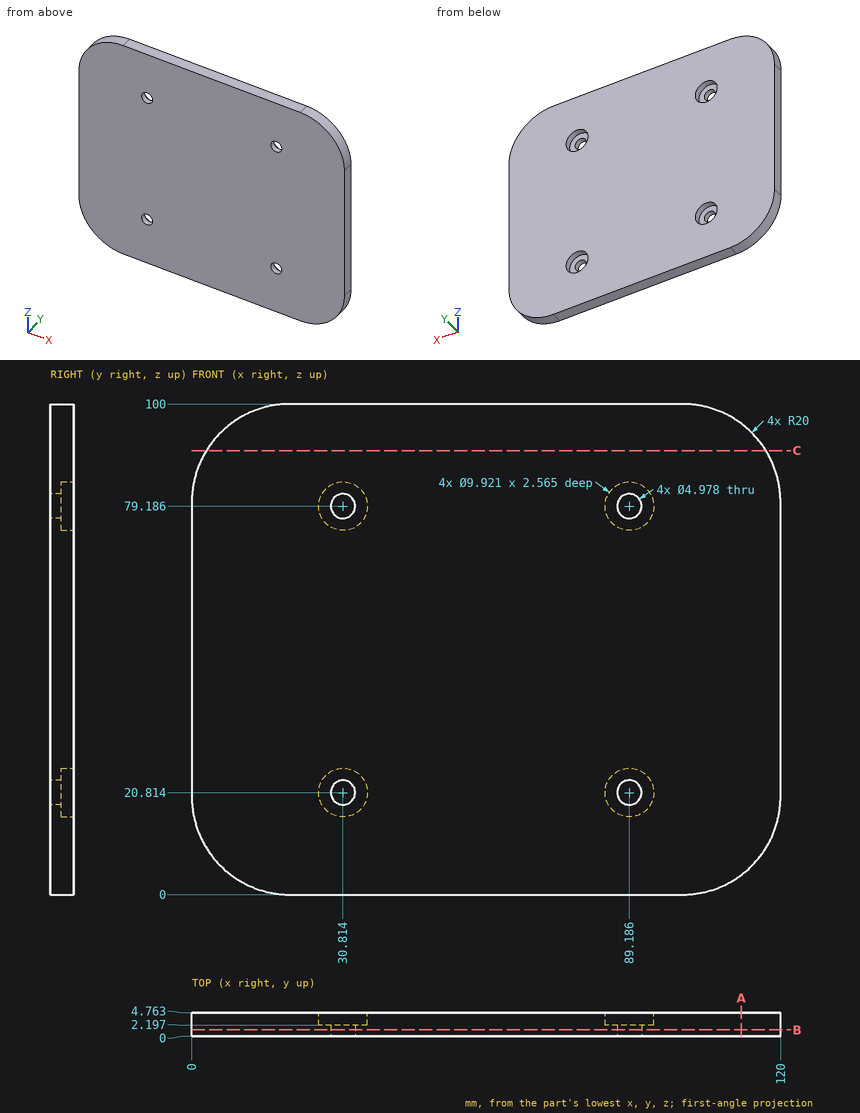
Could you check a few things on this drawing? It's one solid part, dimensions in mm from its lowest x, y, z. Give positions to 0.01 mm unless a question says otherwise; leave off trailing zeros. Write each loop counter-clockwise with the first axis right and the second up, starting at its lowest first coordinate (ties: lowest second). Pieces come first, ordered by that corner, then holes.
(1) Imagine slicing it at C-C, the plane z = 90.5. Write out the boundary of the cut face in (x, y), and give its area (3 significant figures).
Output values:
outline: (2.98, 0) - (117.02, 0) - (117.02, 4.76) - (2.98, 4.76) - close
area: 543 mm2
(2) Imagine slicing it at A-A, the plane x = 112. Write out the boundary of the cut face in (y, z), and give its area (3 significant figures).
Output values:
outline: (0, 4) - (4.76, 4) - (4.76, 96) - (0, 96) - close
area: 438 mm2
(3) If I drill on L1, parallel to X at y = 4, z = 81 (1 decimal); L2, parallel to Z at x = 88, y = 2.3; L3, parallel to X at y = 2.05, z = 91.5 (1 decimal), over which ranges is the centre line in solid material (lowest first)?
Output values:
L1: x = 0 to 26.2, 35.4 to 84.6, 93.8 to 120
L2: z = 0 to 16, 25.63 to 74.37, 84 to 100
L3: x = 3.6 to 116.4
(4) Will these pins go through, and if not, where does the flat tip stop? pin 1 (1.5 mm diameter, centred on y = 1, z = 86, fed in from -X); pin 2 (5.5 mm diameter, centred on x = 89.19, z = 20.81, fed in from +Y); pin 3 (1 mm diameter, centred on x = 13.5, y = 1.5, fed in from +Z).
Output values:
pin 1: stops at x = 0.7
pin 2: stops at y = 2.2
pin 3: stops at z = 99.08
(5) Imagine slicing it at B-B, the plane y = 1.25. Write out the boundary of the cut face in (x, z) (1 decimal).
Output values:
outline: (0, 20) arc R20 ccw to (20, 0) - (100, 0) arc R20 ccw to (120, 20) - (120, 80) arc R20 ccw to (100, 100) - (20, 100) arc R20 ccw to (0, 80) - close; hole circle Ø5 at (30.8, 20.8); hole circle Ø5 at (30.8, 79.2); hole circle Ø5 at (89.2, 20.8); hole circle Ø5 at (89.2, 79.2)
